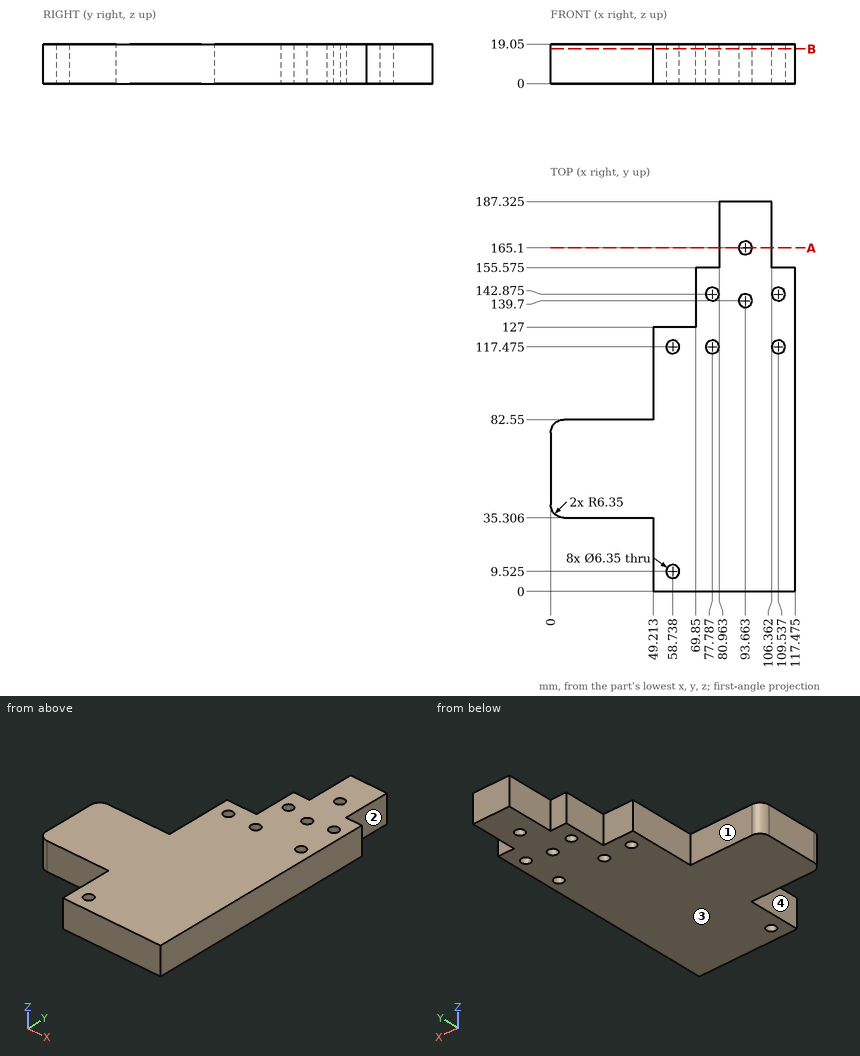
Input: dimensioned drawing with shaded views. Units: mm. Origin: part minimum x, y, z. A direction names the side the tool comes from. Coordinates: 2 decimals unless noted, no trailing zeros. Order: outer loops, then holes, each group sorted by start corner. A loop starts at its lowest first (then second) coordinate and runs counter-clockwise, first axis right, second up.
(1) Material intervals for probe 1 along Y at (x, z) = (77.5, 3.5) (1 decimal); probe 2 along X at (y, z) = (106, 8.5) (1 decimal); probe 3 along Y at (x, z) = (61.5, 15.75), sorted ascending.
(2) Access query for the marked faces 1, 2, 3 and 4. Directions: +Z, -Z, +X, -X, +Y, -Y. A direction counts if a zero-diameter tool reaches every point of the face in a straight line with its end or side. Return the directions, or none.
(3) Section query A-A (y = 165.1). Return the cut outline in (x, z).
(4) First-contact query: pin 1 (5.5 mm diameter, centred on y = 165.5, z = 12, fed in from -X); pin 2 (4 mm diameter, centred on y = 97.5, z = 15, fed in from -X); pin 3 (2 mm diameter, centred on x = 21.5, z = 8, fed in from +Y). Flat tips, straight axial feed; report the tip coordinate or a pass-through.
(5) Section query B-B (z = 16.75). State how many separate pieces and enclosed holes the cut face has, plus the area to 3 significant figures.
Solution:
1. probe 1: y = 0 to 114.3, 120.6 to 139.7, 146 to 155.6
1. probe 2: x = 49.2 to 117.5
1. probe 3: y = 0 to 7.96, 11.09 to 115.91, 119.04 to 127
2. face 1: +Z, -Z, -X, +Y
2. face 2: +Z, -Z, +X, +Y
2. face 3: -Z, +X, -X, +Y, -Y
2. face 4: +Z, -Z, -X, -Y
3. outline: (80.96, 0) - (90.49, 0) - (90.49, 19.05) - (80.96, 19.05) - close; (96.84, 0) - (106.36, 0) - (106.36, 19.05) - (96.84, 19.05) - close
4. pin 1: stops at x = 80.96
4. pin 2: stops at x = 49.21
4. pin 3: stops at y = 82.55
5. separate pieces: 1
5. enclosed holes: 8
5. area: 12,900 mm2
